Geometry check sheet. Reference: the model listing, model coordinates, mm. Face numbers are marked on the shaded views. A direction names the side the tool comes from. Give positions to 0.01 mm unless a question says otherwise; leave off trailing zeros. Loops run counter-clockwise (first coordinate to the right, second up) from the corner with the lowest first, then second, coordinate; pieces in that order, holes last. Notation, with made-up numbers: (27.5, -20.75) -> (51.5, -20.75) arc R27 cw to (51.5, 18.25) -> close; hole circle Ø2 at (35.5, 25.25). An arc over 180 degrees is marked (long way). One line per item, written item: value. Start each with the question number.
(1) Scan lines: line 1 along X through (y, z) = (-0.75, -18.5) (3 decimals); line 2 along Y through (x, z) = (51, 23); line 3 along Z through (x, y) = (32.5, -4.5). Record each from-to range of solid material in increasing order. Write a range as from..to.
(2) Sectioned sample at C-C, the plane y = -10.5. Record the cut outline in (x, z) (3 decimals).
(3) Gauge pin test, flat ends, axial feed: pin 1 Ø4 at (x, y) = (9, -2) entering from +Z; pin 2 Ø6 at (x, z) = (10, 20) entering from -Y (3 decimals); pin 3 Ø5 at (x, y) = (26, -10.5) entering from -Z; pin 4 Ø3 at (x, z) = (7.94, 20.39) entering from +Y. Record the tip position at first contact, or that the pin passes through.
(4) Sectioned sample at A-A, the plane z = 18. Record the cut outline in (x, y) (1 decimal), then the cut area to 3 significant figures.
(5) Sectioned sample at D-D, the plane z = -11.5. Record the cut outline in (x, y).
(6) Tool access check on the marked faces 3, 4 and 5. Record the directions out of +Z, -Z, +X, -X, +Y, -Y that give a thin tool (end or side, any length) a straight path to the whole face; none if there is none.
(7) Sectioned sample at B-B, the plane x = 11.5. Record the cut outline in (y, z) (1 decimal), then the cut area to 3 significant figures.
(8) Draft check along X on the marked faces 1 and 2. Enter one of: pulls with the +X half, pulls with the -X half, needs draft (parallel to the pull), parting line crosses it, or undercut.
from build123d import *

# Parameters (mm, degrees)
SKETCH1_R                = 16.9545
BOSS_EXTRUDE1_DEPTH      = 50.8
SKETCH2_R                = 16.9545
BOSS_EXTRUDE2_DEPTH      = 34.925
SKETCH3_R                = 13.081
CUT_EXTRUDE1_DEPTH       = 50.8
SKETCH5_R                = 13.081
CUT_EXTRUDE2_DEPTH       = 69.85
CUT_EXTRUDE4_DEPTH       = 79.088942658
CUT_EXTRUDE4_DEPTH_BACK  = 79.088942658
SKETCH6_R                = 3.81
BOSS_EXTRUDE3_REACH      = 93.464
BOSS_EXTRUDE3_END_RADIUS = 16.9545
SKETCH8_W                = 15.875
SKETCH8_H                = 5.08
CUT_EXTRUDE5_REACH       = 93.464
CUT_EXTRUDE5_END_RADIUS  = 16.9545
SKETCH9_W                = 12.573
SKETCH9_H                = 1.905
SKETCH10_R               = 1.5875
CUT_EXTRUDE6_DEPTH       = 78.461619779


with BuildPart() as part:
    # Sketch1 → Boss-Extrude1 (new body)
    with BuildSketch(Plane(origin=(0, 0, 0), x_dir=(0, 0, -1), z_dir=(1, 0, 0))):
        Circle(SKETCH1_R)
    extrude(amount=BOSS_EXTRUDE1_DEPTH)

    # Sketch2 → Boss-Extrude2 (add, symmetric)
    with BuildSketch(Plane.XY):
        with Locations((50.8, 0)):
            Circle(SKETCH2_R)
    extrude(amount=BOSS_EXTRUDE2_DEPTH, both=True)

    # Sketch3 → Cut-Extrude1 (cut)
    with BuildSketch(Plane.ZY):
        Circle(SKETCH3_R)
    extrude(amount=-CUT_EXTRUDE1_DEPTH, mode=Mode.SUBTRACT)

    # Sketch5 → Cut-Extrude2 (cut)
    with BuildSketch(Plane(origin=(0, 0, -34.925), x_dir=(-1, 0, 0), z_dir=(0, 0, -1))):
        with Locations((-50.8, 0)):
            Circle(SKETCH5_R)
    extrude(amount=-CUT_EXTRUDE2_DEPTH, mode=Mode.SUBTRACT)

    # Sketch6 → Cut-Extrude4 (cut, two sides: drawn at the far end of the back side and taken through both)
    with BuildSketch(Plane(origin=(0, 0, 0), x_dir=(0, 0, -1), z_dir=(1, 0, 0)).offset(-CUT_EXTRUDE4_DEPTH_BACK)):
        with Locations(Location((0, 0, 0), (0, 0, 180))):
            Circle(SKETCH6_R)
    extrude(amount=CUT_EXTRUDE4_DEPTH + CUT_EXTRUDE4_DEPTH_BACK, mode=Mode.SUBTRACT)

    # SurfaceCut1
    split(bisect_by=Plane(origin=(0, 0, 0), x_dir=(1, 0, 0), z_dir=(0, 1, 0)), keep=Keep.BOTTOM)


with BuildPart() as body_2:
    # Boss-Extrude3: up to this cylinder (the profile starts outside it)
    boss_extrude3_end = Plane(origin=(7.9375, 0, 0), z_dir=(-1, 0, 0)) * Cylinder(BOSS_EXTRUDE3_END_RADIUS, 221.837, mode=Mode.PRIVATE)
    # Sketch8 → Boss-Extrude3 (new, up to the surface)
    with BuildSketch(Plane.XY.offset(24.13), mode=Mode.PRIVATE) as boss_extrude3_sk1:
        with Locations((7.9375, -2.54)):
            Rectangle(SKETCH8_W, SKETCH8_H)
    boss_extrude3_tool1 = extrude(boss_extrude3_sk1.sketch, amount=-BOSS_EXTRUDE3_REACH, mode=Mode.PRIVATE) - boss_extrude3_end
    add(boss_extrude3_tool1.solids().sort_by_distance((7.9375, -2.54, 24.13))[0])

    # Cut-Extrude5: up to this cylinder (the profile starts outside it)
    cut_extrude5_end = Plane(origin=(7.9375, 0, 0), z_dir=(-1, 0, 0)) * Cylinder(CUT_EXTRUDE5_END_RADIUS, 221.837, mode=Mode.PRIVATE)
    # Sketch9 → Cut-Extrude5 (cut, up to the surface)
    with BuildSketch(Plane.XY.offset(24.13), mode=Mode.PRIVATE) as cut_extrude5_sk1:
        with Locations((7.9375, -4.1275)):
            Rectangle(SKETCH9_W, SKETCH9_H)
    cut_extrude5_tool1 = extrude(cut_extrude5_sk1.sketch, amount=-CUT_EXTRUDE5_REACH, mode=Mode.PRIVATE) - cut_extrude5_end
    add(cut_extrude5_tool1.solids().sort_by_distance((7.9375, -4.1275, 24.13))[0], mode=Mode.SUBTRACT)


with BuildPart() as body_3:
    # Mirror1: mirrored copy
    add(body_2.part.mirror(Plane.XY))


with BuildPart() as part_1:
    add(part.part)

    # Intersect1: read off the stored shape, not the designer's step
    # Intersect1: union body 3, body 2
    add(body_3.part)
    add(body_2.part)

    # Sketch10 → Cut-Extrude6 (cut, through all)
    with BuildSketch(Plane.XZ.offset(3.175)):
        with Locations(Location((7.9375, 20.392281148, 0), (0, 0, 270))):
            Circle(SKETCH10_R)
    cut_extrude6 = extrude(amount=-CUT_EXTRUDE6_DEPTH, mode=Mode.SUBTRACT)

    # Mirror2: Cut-Extrude6 across plane
    add(cut_extrude6.mirror(Plane.XY), mode=Mode.SUBTRACT)


solid = part_1.part
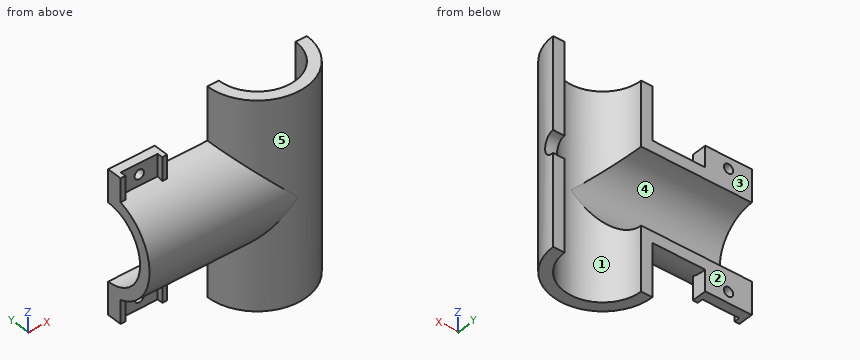
Calculated:
1. line 1: x = 0..15.875, 33.862..37.741, 63.859..67.738
1. line 2: y = -16.95..-13.08
1. line 3: z = -16.35..-12.28, 12.28..16.35
2. outline: (0, -13.312) -> (37.488, -13.312) -> (37.488, -34.925) -> (42.999, -34.925) -> (42.999, -7.801) -> (0, -7.801) -> close; (0, 7.801) -> (42.999, 7.801) -> (42.999, 34.925) -> (37.488, 34.925) -> (37.488, 13.312) -> (0, 13.312) -> close; (58.601, -34.925) -> (64.112, -34.925) -> (64.112, 34.925) -> (58.601, 34.925) -> close
3. pin 1: stops at z = 24.13
3. pin 2: stops at y = -3.175
3. pin 3: stops at z = -14.95
3. pin 4: passes through
4. outline: (0, -5.1) -> (1.7, -5.1) -> (1.7, -3.2) -> (14.2, -3.2) -> (14.2, -5.1) -> (15.9, -5.1) -> (15.9, 0) -> (0, 0) -> close; (33.8, 0) arc R17 ccw to (67.8, 0) -> (63.9, 0) arc R13.1 cw to (37.7, 0) -> close
4. area: 239 mm2
5. outline: (0, -12.46) -> (39.3, -12.46) arc R16.95 ccw to (67.75, 0) -> (63.88, 0) arc R13.08 cw to (39.3, -6.23) -> (0, -6.23) -> close
6. face 3: +Z, -Z, +X, -X, +Y
6. face 4: -X, +Y
6. face 5: -Y
7. outline: (-3.2, -24.1) -> (0, -24.1) -> (0, -13.1) arc R13.1 cw to (0, 13.1) -> (0, 24.1) -> (-3.2, 24.1) -> (-3.2, 16.7) arc R17 ccw to (-3.2, -16.7) -> close
7. area: 229 mm2
8. face 1: undercut
8. face 2: needs draft
